Verification items for the finished model (mm, model axes). Face numbers are marked on the shaded views. A direction names the side the tool comes from. Coordinates: 2 decimals unless noted, no trailing zeros. One line per item, written item: value.
Autodesk Inventor part; units mm, degrees
ref_plane "YZ Plane" through (0, 0, 0) normal (1, 0, 0) x (0, 1, 0)
ref_plane "XZ Plane" through (0, 0, 0) normal (0, 1, 0) x (-1, 0, 0)
ref_plane "XY Plane" through (0, 0, 0) normal (0, 0, 1) x (1, 0, 0)
sketch "Sketch1" plane through (0, 0, 0) normal (0, 0, 1) x (1, 0, 0)
  circle A0 centre (0, 0) radius 9.525
  circle A1 centre (0, 0) radius 17.4625
  line L0 (-31.75, 31.75) -> (31.75, 31.75)
  line L1 (31.75, 31.75) -> (31.75, -31.75)
  line L2 (31.75, -31.75) -> (-31.75, -31.75)
  line L3 (-31.75, -31.75) -> (-31.75, 31.75)
  line L4 (-31.75, 0) -> (31.75, 0) construction
  line L5 (0, 31.75) -> (0, -31.75) construction
  circle A2 centre (0, 25.4) radius 2.3495
  circle A3 centre (-25.4, 0) radius 2.3495
  circle A4 centre (25.4, 0) radius 2.3495
  circle A5 centre (0, -25.4) radius 2.3495
  line L6 (-27.0002, 27.0002) -> (27.0002, 27.0002) construction
  line L7 (27.0002, 27.0002) -> (27.0002, -27.0002) construction
  line L8 (27.0002, -27.0002) -> (-27.0002, -27.0002) construction
  line L9 (-27.0002, -27.0002) -> (-27.0002, 27.0002) construction
  circle A6 centre (-25.0002, 25.0002) radius 2 construction
  circle A7 centre (25.0002, 25.0002) radius 2 construction
  circle A8 centre (25.0002, -25.0002) radius 2 construction
  circle A9 centre (-25.0002, -25.0002) radius 2 construction
  circle A10 centre (0, 25.4) radius 3.81
  circle A11 centre (25.4, 0) radius 3.81
  circle A12 centre (-25.4, 0) radius 3.81
  circle A13 centre (0, -25.4) radius 3.81
  arc A14 (-24.3637, -3.6664) -> (-3.6664, -24.3637) centre (0, 0) ccw
  arc A15 (3.6664, -24.3637) -> (24.3637, -3.6664) centre (0, 0) ccw
  arc A16 (24.3637, 3.6664) -> (3.6664, 24.3637) centre (0, 0) ccw
  arc A17 (-3.6664, 24.3637) -> (-24.3637, 3.6664) centre (0, 0) ccw
  circle A18 centre (-25.0002, 25.0002) radius 2.1209
  circle A19 centre (25.0002, 25.0002) radius 2.1209
  circle A20 centre (25.0002, -25.0002) radius 2.1209
  circle A21 centre (-25.0002, -25.0002) radius 2.1209
  point P0 (0, 27.0002)
  point P1 (-27.0002, 0)
  dimension "d0" = 19.05
  dimension "d2" = 63.5
  dimension "d3" = 63.5
  dimension "d4" = 4.699
  dimension "d6" = 25.4
  dimension "d7" = 25.4
  dimension "d8" = 25.4
  dimension "d9" = 25.4
  dimension "d10" = 34.925
  dimension "d13" = 54.0004
  dimension "d14" = 54.0004
  dimension "d15" = 4
  dimension "d16" = 24.638
  dimension "d17" = 7.62
  dimension "d26" = 4.2418
extrude "Extrusion1" add sketch "Sketch1" against normal blind 22.9108 contours A1 | L0 L1 L2 L3 | A10 | A10 A16 A11 A15 A13 A14 A12 A17 | A12 | A11 | A13
extrude "Extrusion2" cut sketch "Sketch1" against normal blind 12.7 contours A1 | A10 | A12 | A11 | A13
extrude "Extrusion3" add sketch "Sketch1" along normal blind 3 contours A10 A16 A11 A15 A13 A14 A12 A17
fillet "Fillet1" radius 6.35 4 edges at (-31.75, 31.75, -11.4554) (31.75, 31.75, -11.4554) (-31.75, -31.75, -11.4554) (31.75, -31.75, -11.4554)
chamfer "Chamfer1" distance 0.635 angle 45 6 edges at (-17.4625, 0, 3) (-9.525, 0, -22.9108) (17.4217, -17.4217, 3) (-17.4217, -17.4217, 3) (-17.4217, 17.4217, 3) (17.4217, 17.4217, 3)
thread "Thread1"
thread "Thread2"
thread "Thread3"
thread "Thread4"
sketch "Sketch2" plane through (-25.4, -31.75, 0) normal (0, -1, 0) x (1, 0, 0)
  line L0 (50.8, -22.9108) -> (0, -22.9108)
  line L1 (7.8994, -6.35) -> (42.9006, -6.35) construction
  circle A0 centre (7.8994, -6.35) radius 3.175
  circle A1 centre (42.9006, -6.35) radius 3.175
  line L2 (25.4, -22.9108) -> (25.4, 0) construction
  point P0 (25.4, -6.35)
  dimension "d35" = 35.0012
  dimension "d37" = 6.35
  dimension "d38" = 16.5608
extrude "Extrusion4" cut sketch "Sketch2" against normal blind 12.7
sketch "Sketch3" plane through (-25.4, 31.75, 0) normal (0, 1, 0) x (1, 0, 0)
  line L0 (0, 22.9108) -> (50.8, 22.9108)
  line L1 (0, 0) -> (50.8, 0)
  line L2 (7.8994, 6.35) -> (42.9006, 6.35) construction
  line L3 (25.4, 22.9108) -> (25.4, 0) construction
  circle A0 centre (7.8994, 6.35) radius 3.175
  circle A1 centre (42.9006, 6.35) radius 3.175
  point P0 (25.4, 6.35)
  dimension "d41" = 6.35
  dimension "d43" = 16.5608
  dimension "d44" = 35.0012
extrude "Extrusion5" cut sketch "Sketch3" against normal blind 12.7
thread "Thread5"
thread "Thread6"
thread "Thread7"
thread "Thread8"
properties part number "P80 Motor Block" material "Steel"
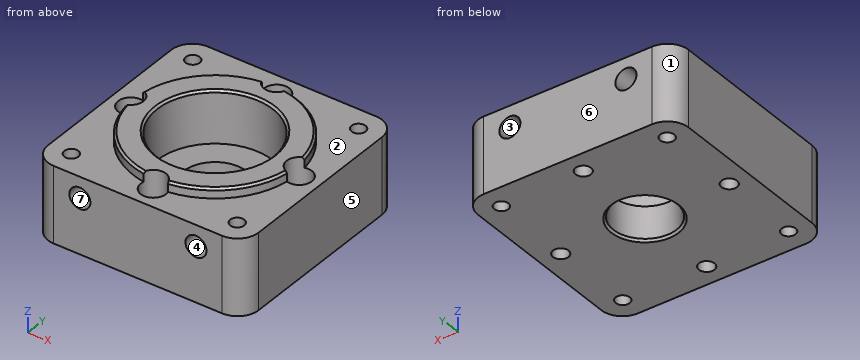
Item 1: Access from +Z, -Z, +X, -X, +Y, -Y to the whole of each face (thin tool, end or side, straight path). Record for the marked faces 1, 2, 3 and 4.
The answers:
face 1: +Z, -Z, -X, +Y
face 2: +Z
face 3: +Y
face 4: -Y
Item 2: Cross-section at A-A, the plane x = 0. Give the number of separate pieces and of enclosed holes in the cut face, and give its area (3 significant figures).
The answers:
separate pieces: 4
enclosed holes: 0
area: 551 mm²
Item 3: Draft check along X on the marked faces 5, 6 and 7. Enter one of: released by +X, released by -X, zero draft, split by the parting line, or undercut.
The answers:
face 5: released by +X
face 6: zero draft
face 7: undercut
Item 4: Go/stop test with flat-tipped pins: P1, Ø21, axis at x = 0, y = 0, coming from the +Z side; P2, Ø10, axis at x = -22.5, y = 22.5, coming from the +Z side; P3, Ø5.5, axis at x = -17.5, z = -6.35, coming from the -Y side. Record where each tip stops, or that it passes through.
The answers:
P1: stops at z = -12.7
P2: stops at z = 0
P3: stops at y = -19.05
Item 5: Scan lines: line 1 (X direction, y = 23.5, z = -0.5); line 2 (X direction, y = 1, z = -14.75); line 3 (Y direction, x = 25.5, z = -9.25). Record each from-to range of solid material in increasing order.
The answers:
line 1: x = -31.75 to -26.5, -23.5 to -3.3, 3.3 to 23.5, 26.5 to 31.75
line 2: x = -31.75 to -27.53, -23.27 to -9.47, 9.47 to 23.27, 27.53 to 31.75
line 3: y = -31.75 to -27.06, -22.94 to -3.81, 3.81 to 22.94, 27.06 to 31.75
